Verification items for the finished model (mm, model axes). A direction names the side the tool comes from. Round coordinates to 2 decimals unless told otherwise and drop trailing zeros. Loops run counter-clockwise (first coordinate to the right, second up) from the corner with the lowest first, then second, coordinate; pieces in that order, holes last. Notation, with made-up numbers: M -14.75,-39.75 L 42.25,-39.75 A19 cw 42.25,-23.75 Z; hole C 88.25,15 d3. An arc over 180 degrees is marked long. One line per item, written item: value.
Autodesk Inventor part; units mm, degrees
ref_plane "YZ Plane" through (0, 0, 0) normal (1, 0, 0) x (0, 1, 0)
ref_plane "XZ Plane" through (0, 0, 0) normal (0, 1, 0) x (-1, 0, 0)
ref_plane "XY Plane" through (0, 0, 0) normal (0, 0, 1) x (1, 0, 0)
sketch "Sketch2" plane through (0, 0, 0) normal (0, 0, 1) x (1, 0, 0)
  line L0 (0, 0) -> (4.8, 0)
  line L1 (4.8, 0) -> (4.8, 25)
  line L2 (4.8, 25) -> (0, 25)
  line L3 (0, 25) -> (0, 0)
  dimension "d11" = 25
  dimension "d12" = 4.8
extrude "Extrusion2" add sketch "Sketch2" along normal mid plane 45
sketch "Sketch3" plane through (0, 0, 22.5) normal (0, 0, 1) x (1, 0, 0)
  line L0 (4.8, 0) -> (4.8, 25)
  line L1 (4.8, 25) -> (44.8, 25)
  line L2 (44.8, 25) -> (45.7352, 3.5814) construction
  line L3 (45.7352, 3.5814) -> (4.8, 0)
  arc A0 (45.7352, 3.5814) -> (44.8, 25) centre (44.8, 14.2703) ccw
  line L4 (46.55, 17.3014) -> (43.05, 11.2392) construction
  line L5 (44.3849, 18.5514) -> (40.8849, 12.4892)
  line L6 (45.2151, 9.9892) -> (48.7151, 16.0514)
  arc A1 (48.7151, 16.0514) -> (44.3849, 18.5514) centre (46.55, 17.3014) ccw
  arc A2 (40.8849, 12.4892) -> (45.2151, 9.9892) centre (43.05, 11.2392) ccw
  point P0 (0, 0)
  dimension "d15" = 40
  dimension "d16" = 85
  dimension "d17" = 5
  dimension "d18" = 7
  dimension "d19" = 30
extrude "Extrusion3" add sketch "Sketch3" against normal blind 3
mirror "Mirror1" about plane through (0, 0, 0) normal (0, 0, 1) of "Extrusion3"
chamfer "Chamfer1" distance 2 angle 45 2 edges at (4.8, 12.5, 19.5) (4.8, 12.5, -19.5)
properties part number "Solder Roll Support 2" material "SAE 1020"
(1) Sectioned sample at C-C on x = 43.05. Enter the section's corners in (y, z).
Completed:
outline: M 3.35,-22.5 L 8.74,-22.5 L 8.74,-19.5 L 3.35,-19.5 Z; M 3.35,19.5 L 8.74,19.5 L 8.74,22.5 L 3.35,22.5 Z; M 16.24,-22.5 L 25,-22.5 L 25,-19.5 L 16.24,-19.5 Z; M 16.24,19.5 L 25,19.5 L 25,22.5 L 16.24,22.5 Z
(2) Sectioned sample at D-D on z = 2. Enter the section's corners in (x, y).
Completed:
outline: M 0,0 L 4.8,0 L 4.8,25 L 0,25 Z
(3) Depth check by flat-ended pin: pin 1 Ø4 at (y, z) = (8, 3) entering from +X. Enter the tip coordinate at first touch or a pass-through.
Completed:
pin 1: stops at x = 4.8
(4) Thickness scan on L1, parallel to Z at x = 52, y = 9.5; L2, parallel to X at y = 3, z = -13.5; L3, parallel to Z at x = 5, y = 18.25. Record the ranges inside material, lowest first. Write a range as from..to.
Completed:
L1: z = -22.5..-19.5, 19.5..22.5
L2: x = 0..4.8
L3: z = -22.5..-17.7, 17.7..22.5
(5) Sectioned sample at A-A on x = 36. Enter the section's corners in (y, z), and give its area (3 significant figures).
Completed:
outline: M 2.73,-22.5 L 25,-22.5 L 25,-19.5 L 2.73,-19.5 Z; M 2.73,19.5 L 25,19.5 L 25,22.5 L 2.73,22.5 Z
area: 134 mm^2
(6) Sectioned sample at B-B on y = 13.75. Enter the section's corners in (x, z).
Completed:
outline: M 0,-22.5 L 41.61,-22.5 L 41.61,-19.5 L 6.8,-19.5 L 4.8,-17.5 L 4.8,17.5 L 6.8,19.5 L 41.61,19.5 L 41.61,22.5 L 0,22.5 Z; M 47.39,-22.5 L 55.52,-22.5 L 55.52,-19.5 L 47.39,-19.5 Z; M 47.39,19.5 L 55.52,19.5 L 55.52,22.5 L 47.39,22.5 Z
(7) Tool access check on faces 1 (the face through (42.61, 15.48, -21.02)), 2 (the face through (4.8, 12, 0)), 3 (the face through (55.507, 14.967, -21.021)). Record the directions out of +Z, -Z, +X, -X, +Y, -Y that give a thin tool (end or side, any length) a straight path to the whole face; none if there is none.
Completed:
face 1: +Z, -Z
face 2: +X, +Y, -Y
face 3: +Z, -Z, +X
(8) Mould release check, pull along X, two halves, no side actions. Record for faces 4 (the face through (42.66, 15.56, 21.02)), 5 (the face through (0, 13, 0)), 6 (the face through (5.8, 12.3, -18.5)): +X half, -X half, draft (parallel to the pull), parting line (faces both ways), or undercut.
Completed:
face 4: undercut
face 5: -X half
face 6: +X half
